Answer from the drawing. Dimensions are ordinates in mm from the lowest x, y and z of the part. A direction names the side the tool comes from. Round coordinates to 2 decimals unless told otherwise and drop trailing zeros. Write each loop counter-clockwise with the first axis right and the second up, starting at its lowest first coordinate (ties: lowest second). Pieces come first, ordered by that corner, then holes.
1. A flat-ended cylindrical pin translates along its axis: pin 1 Ø4 at (x, z) = (48.5, 10.5) entering from -Y. Find the tip coordinate at first contact, or state that the pin passes through.
2. Find section A-A (z = 7.5). Write down the section's boundary in (x, y).
3. Determine the mould class of the marked faces 1, 2, 3 and 4 for opening direction X: pulls with the +X half, pulls with the -X half, needs draft (parallel to the pull), parting line crosses it, or undercut.
4. Find section B-B (x = 40). Write down the section's boundary in (y, z), and give its area (4 significant figures).
5. Straight lines are drawn through the part: probe 1 along Z at (x, y) = (27.5, 13.75); probe 2 along Y at (x, z) = (40, 10.75); probe 3 along X at (y, z) = (7, 4). For each, find the intervals that lie inside material, in ascending order.
6. Find section D-D (x = 72.5). Write down the section's boundary in (y, z), and give its area (3 significant figures).
7. A tool of negligible diameter and unlimited length cuts with its end or side. For the marked faces 5 and 6, from which of +Z, -Z, +X, -X, +Y, -Y can it reach the whole face along a straight path? Write none if from no direction.
8. Find section C-C (z = 2.75). Write down the section's boundary in (x, y), and give its area (3 significant figures).
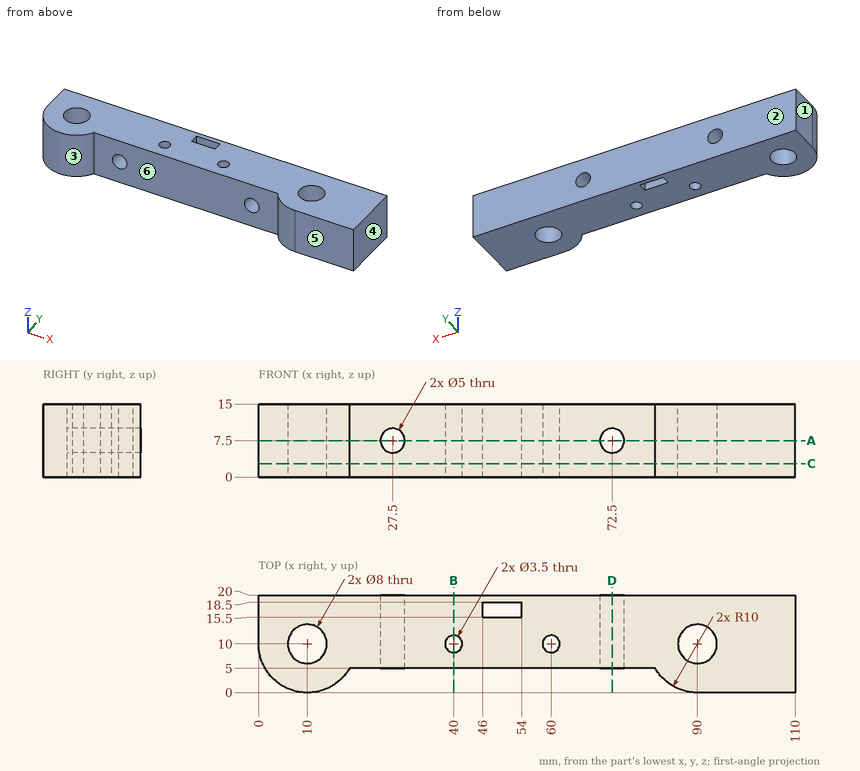
Worked answers:
1. pin 1: stops at y = 5
2. outline: (0, 10) arc R10 ccw to (18.66, 5) - (25, 5) - (25, 20) - (0, 20) - close; (30, 5) - (70, 5) - (70, 20) - (30, 20) - close; (75, 5) - (81.34, 5) arc R10 ccw to (90, 0) - (110, 0) - (110, 20) - (75, 20) - close; hole circle Ø8 at (10, 10); hole circle Ø3.5 at (40, 10); hole (46, 15.5) - (54, 15.5) - (54, 18.5) - (46, 18.5) - close; hole circle Ø3.5 at (60, 10); hole circle Ø8 at (90, 10)
3. face 1: pulls with the -X half
3. face 2: needs draft
3. face 3: undercut
3. face 4: pulls with the +X half
4. outline: (5, 0) - (8.25, 0) - (8.25, 15) - (5, 15) - close; (11.75, 0) - (20, 0) - (20, 15) - (11.75, 15) - close
4. area: 172.5 mm2
5. probe 1: z = 0 to 5, 10 to 15
5. probe 2: y = 5 to 8.25, 11.75 to 20
5. probe 3: x = 0.46 to 7.35, 12.65 to 87.35, 92.65 to 110
6. outline: (5, 0) - (20, 0) - (20, 5) - (5, 5) - close; (5, 10) - (20, 10) - (20, 15) - (5, 15) - close
6. area: 150 mm2
7. face 5: +Z, -Z, +X, -X, -Y
7. face 6: +Z, -Z, -Y
8. outline: (0, 10) arc R10 ccw to (18.66, 5) - (81.34, 5) arc R10 ccw to (90, 0) - (110, 0) - (110, 20) - (0, 20) - close; hole circle Ø8 at (10, 10); hole circle Ø3.5 at (40, 10); hole (46, 15.5) - (54, 15.5) - (54, 18.5) - (46, 18.5) - close; hole circle Ø3.5 at (60, 10); hole circle Ø8 at (90, 10)
8. area: 1,700 mm2
